Could you check a few things on this model? Use its own coordinates, in mm. A direction names the side the tool comes from. Round coordinates to 2 decimals unless told otherwise and drop trailing zeros. Loops run counter-clockwise (first coordinate to the right, second up) from the corner with the lowest first, then second, coordinate; pieces in that order, holes last. Notation, with made-up numbers: (24.5, -31) - (76.5, -31) arc R19 cw to (76.5, -23) - close; hole circle Ø7 at (13, -29.75). An arc over 180 degrees is marked (long way). Answer as CSV lines item,"result". Start each with the question number.
1) Suppose I cut it at D-D, the plane x = 17. Write out the boundary of the cut face in (y, z).
2) Which directions (+Z, -Z, +X, -X, +Y, -Y) give clear straight access to the entire face, cutting with the end or side of a thin tool? Please do faces 4 (the face through (14.9, 38, 1.5)), 5 (the face through (41.135, 38.66, 1.479)), 6 (the face through (18, 22, 1)).
3) I'm going to push flat-ended pins straight in: pin 1 Ø1 at (y, z) = (20.5, 2) entering from -X; pin 2 Ø1.6 at (y, z) = (20, 1.5) entering from +X; pin 3 Ø1.5 at (y, z) = (36, 1) entering from -X. Where does each tip first touch, or does it pass through?
4) We'd pull the mould along X, two halves only. Please class faces 1 (the face through (38.69, 41.165, 1.479)), 2 (the face through (5, 14.9, 1.5)), 3 (the face through (15, 28, 0)): pulls with the +X half, pulls with the -X half, needs draft (parallel to the pull), parting line crosses it, or undercut.
5) Suppose I cut it at B-B, the plane y = 19.5. Write out the boundary of the cut face in (x, z), then the cut area to 3 significant figures.
6) Suppose I cut it at C-C, the plane x = 32.5. Write out the boundary of the cut face in (y, z).
7) Please list where these lines run through material, in increasing order: line 1 along Y through (x, z) = (2.5, 1.25); line 2 along X through (y, z) = (5, 0.65); line 3 along X through (y, z) = (31.5, 0.2).
8) Suppose I cut it at A-A, the plane y = 2. Write out the boundary of the cut face in (x, z).
```python
from build123d import *

# Parameters (mm, degrees)
BOSS_EXTRUDE1_DEPTH = 3
CUT_EXTRUDE1_DEPTH  = 10
SKETCH3_OUTSIDE_W   = 98.222
SKETCH3_OUTSIDE_H   = 98.222
CUT_EXTRUDE2_DEPTH  = 10
SKETCH5_R           = 7.5
CUT_EXTRUDE3_DEPTH  = 1
CUT_EXTRUDE4_DEPTH  = 2


with BuildPart() as part:
    # Sketch1 → Boss-Extrude1 (new body)
    with BuildSketch(Plane.XY):
        with BuildLine():
            ThreePointArc((59, 21.5), (35.850628714, 56.145482469), (-5.016504294, 48.016504294))
            Line((-5.016504294, 48.016504294), (48.016504294, -5.016504294))
            ThreePointArc((48.016504294, -5.016504294), (56.145482469, 7.149371286), (59, 21.5))
        make_face()
        with BuildLine():
            Line((48.016504294, -5.016504294), (-5.016504294, 48.016504294))
            ThreePointArc((-5.016504294, 48.016504294), (-5.016504294, -5.016504294), (48.016504294, -5.016504294))
        make_face()
    extrude(amount=BOSS_EXTRUDE1_DEPTH)

    # Sketch2 → Cut-Extrude1 (cut)
    with BuildSketch(Plane(origin=(0, 0, 0), x_dir=(-1, 0, 0), z_dir=(0, 0, -1))):
        with BuildLine():
            Line((-40.089276695, 37.614402961), (-42.210597039, 39.735723305))
            ThreePointArc((-42.210597039, 39.735723305), (-42.210597039, 42.210597039), (-39.735723305, 42.210597039))
            Line((-39.735723305, 42.210597039), (-37.614402961, 40.089276695))
            ThreePointArc((-37.614402961, 40.089276695), (-37.614402961, 37.614402961), (-40.089276695, 37.614402961))
        make_face()
        with BuildLine():
            Line((-5.385597039, 40.089276695), (-3.264276695, 42.210597039))
            ThreePointArc((-3.264276695, 42.210597039), (-0.789402961, 42.210597039), (-0.789402961, 39.735723305))
            Line((-0.789402961, 39.735723305), (-2.910723305, 37.614402961))
            ThreePointArc((-2.910723305, 37.614402961), (-5.385597039, 37.614402961), (-5.385597039, 40.089276695))
        make_face()
        with BuildLine():
            Line((-42.033820344, 3.441053391), (-40.266053391, 5.208820344))
            ThreePointArc((-40.266053391, 5.208820344), (-37.791179656, 5.208820344), (-37.791179656, 2.733946609))
            Line((-37.791179656, 2.733946609), (-39.558946609, 0.966179656))
            ThreePointArc((-39.558946609, 0.966179656), (-42.033820344, 0.966179656), (-42.033820344, 3.441053391))
        make_face()
        with BuildLine():
            Line((-3.441053391, 0.966179656), (-5.208820344, 2.733946609))
            ThreePointArc((-5.208820344, 2.733946609), (-5.208820344, 5.208820344), (-2.733946609, 5.208820344))
            Line((-2.733946609, 5.208820344), (-0.966179656, 3.441053391))
            ThreePointArc((-0.966179656, 3.441053391), (-0.966179656, 0.966179656), (-3.441053391, 0.966179656))
        make_face()
    extrude(amount=-CUT_EXTRUDE1_DEPTH, mode=Mode.SUBTRACT)

    # Sketch3 outside → Cut-Extrude2 (cut)
    with BuildSketch(Plane(origin=(0, 0, 0), x_dir=(-1, 0, 0), z_dir=(0, 0, -1))):
        with Locations((-21.5, 21.5)):
            Rectangle(SKETCH3_OUTSIDE_W, SKETCH3_OUTSIDE_H)
        with BuildLine():
            Line((-34.962752532, 44.862247468), (-21.5, 31.399494937))
            Line((-21.5, 31.399494937), (-8.037247468, 44.862247468))
            ThreePointArc((-8.037247468, 44.862247468), (1.862247468, 44.862247468), (1.862247468, 34.962752532))
            Line((1.862247468, 34.962752532), (-11.600505063, 21.5))
            Line((-11.600505063, 21.5), (1.862247468, 8.037247468))
            ThreePointArc((1.862247468, 8.037247468), (1.862247468, -1.862247468), (-8.037247468, -1.862247468))
            Line((-8.037247468, -1.862247468), (-21.5, 11.600505063))
            Line((-21.5, 11.600505063), (-34.962752532, -1.862247468))
            ThreePointArc((-34.962752532, -1.862247468), (-44.862247468, -1.862247468), (-44.862247468, 8.037247468))
            Line((-44.862247468, 8.037247468), (-31.399494937, 21.5))
            Line((-31.399494937, 21.5), (-44.862247468, 34.962752532))
            ThreePointArc((-44.862247468, 34.962752532), (-44.862247468, 44.862247468), (-34.962752532, 44.862247468))
        make_face(mode=Mode.SUBTRACT)
    extrude(amount=-CUT_EXTRUDE2_DEPTH, mode=Mode.SUBTRACT)

    # Sketch5 → Cut-Extrude3 (cut)
    with BuildSketch(Plane(origin=(0, 0, 0), x_dir=(-1, 0, 0), z_dir=(0, 0, -1))):
        with Locations((-21.5, 21.5)):
            Circle(SKETCH5_R)
    extrude(amount=-CUT_EXTRUDE3_DEPTH, mode=Mode.SUBTRACT)

    # Sketch6 → Cut-Extrude4 (cut)
    with BuildSketch(Plane(origin=(0, 0, 1), x_dir=(-1, 0, 0), z_dir=(0, 0, -1))):
        with BuildLine():
            Line((-23.25, 17.5), (-23.25, 25.5))
            ThreePointArc((-23.25, 25.5), (-21.5, 27.25), (-19.75, 25.5))
            Line((-19.75, 25.5), (-19.75, 17.5))
            ThreePointArc((-19.75, 17.5), (-21.5, 15.75), (-23.25, 17.5))
        make_face()
    extrude(amount=-CUT_EXTRUDE4_DEPTH, mode=Mode.SUBTRACT)


solid = part.part
```
Filled sheet:
1,outline,"(7.1, 0) - (15.5, 0) - (15.5, 1) - (27.5, 1) - (27.5, 0) - (35.9, 0) - (35.9, 3) - (7.1, 3) - close"
2,face 4,"+Z, -Z, +Y"
2,face 5,"+Z, -Z"
2,face 6,"-Z"
3,pin 1,"x = 10.1"
3,pin 2,"x = 33.7"
3,pin 3,"x = -3.16"
4,face 1,"undercut"
4,face 2,"pulls with the -X half"
4,face 3,"needs draft"
5,outline,"(9.6, 0) - (14.27, 0) - (14.27, 1) - (19.75, 1) - (19.75, 3) - (9.6, 3) - close; (23.25, 1) - (28.73, 1) - (28.73, 0) - (33.4, 0) - (33.4, 3) - (23.25, 3) - close"
5,area,"49.9 mm²"
6,outline,"(0.6, 0) - (20.4, 0) - (20.4, 3) - (0.6, 3) - close; (22.6, 0) - (42.4, 0) - (42.4, 3) - (22.6, 3) - close"
7,line 1,"-3.89 to 0.48, 4.97 to 12.4, 30.6 to 38.03, 42.66 to 46.89"
7,line 2,"-3.65 to 2.53, 5.39 to 14.9, 28.1 to 37.61, 40.47 to 46.65"
7,line 3,"1.6 to 21.4, 21.6 to 41.4"
8,outline,"(-3.83, 0) - (0.47, 0) - (0.47, 3) - (-3.83, 3) - close; (4.47, 0) - (11.9, 0) - (11.9, 3) - (4.47, 3) - close; (31.1, 0) - (38.53, 0) - (38.53, 3) - (31.1, 3) - close; (42.53, 0) - (46.83, 0) - (46.83, 3) - (42.53, 3) - close"
